```python
from build123d import *

# Parameters (mm, degrees)
MODEL_R             = 14.351
MODEL_R_2           = 2.413
BOSS_EXTRUDE1_DEPTH = 7.874
SKETCH17_R          = 2.0701
CUT_EXTRUDE1_DEPTH  = 8.874
SKETCH18_R          = 2.0193
CUT_EXTRUDE2_DEPTH  = 8.874


with BuildPart() as part:
    # Model → Boss-Extrude1 (new body)
    with BuildSketch(Plane.XY):
        with BuildLine():
            Line((127.809114586, 137.689660276), (-200.005250584, 313.419470721))
            ThreePointArc((-200.005250584, 313.419470721), (-219.438743814, 318.210854709), (-236.308771814, 307.439588539))
            Line((-236.308771814, 307.439588539), (-425.925316767, 28.829603592))
            ThreePointArc((-425.925316767, 28.829603592), (-430.312243104, 13.671313347), (-424.900993017, -1.152223962))
            Line((-424.900993017, -1.152223962), (-385.581467186, -51.204797614))
            ThreePointArc((-385.581467186, -51.204797614), (-376.711879358, -58.358090396), (-365.607528193, -60.913979882))
            Line((-365.607528193, -60.913979882), (-324.737451002, -60.913979882))
            ThreePointArc((-324.737451002, -60.913979882), (-318.798508014, -59.439796386), (-314.23831963, -55.359484793))
            Line((-314.23831963, -55.359484793), (-212.899365952, 93.541257838))
            ThreePointArc((-212.899365952, 93.541257838), (-203.778989185, 101.701881024), (-191.901103209, 104.650248016))
            Line((-191.901103209, 104.650248016), (48.661197018, 104.650248016))
            ThreePointArc((48.661197018, 104.650248016), (64.032332507, 99.471232012), (73.135172194, 86.046168785))
            Line((73.135172194, 86.046168785), (86.727013732, 37.098218434))
            ThreePointArc((86.727013732, 37.098218434), (106.362581421, 15.501750179), (127.326236921, 35.811553418))
            Line((127.326236921, 35.811553418), (140.807890588, 110.809453484))
            ThreePointArc((140.807890588, 110.809453484), (138.675228362, 126.361225539), (127.809114586, 137.689660276))
        make_face()
        with Locations((-323.775189267, -35.513979882)):
            Circle(MODEL_R, mode=Mode.SUBTRACT)
        with Locations((-399.975189267, 2.586020118)):
            Circle(MODEL_R, mode=Mode.SUBTRACT)
        with Locations((107.006236921, 23.111553418)):
            Circle(MODEL_R_2, mode=Mode.SUBTRACT)
        with Locations((94.306236921, 35.811553418)):
            Circle(MODEL_R_2, mode=Mode.SUBTRACT)
        Polygon((110.67241113, 42.161553418), (114.33858534, 35.811553418), (110.67241113, 29.461553418), (103.340062712, 29.461553418), (99.673888502, 35.811553418), (103.340062712, 42.161553418), (107.006236921, 42.161553418), align=None, mode=Mode.SUBTRACT)
        with Locations((119.706236921, 35.811553418)):
            Circle(MODEL_R_2, mode=Mode.SUBTRACT)
        with Locations((107.006236921, 48.511553418)):
            Circle(MODEL_R_2, mode=Mode.SUBTRACT)
        with Locations((-190.707148919, 138.516914683)):
            Circle(MODEL_R, mode=Mode.SUBTRACT)
        with Locations((-178.846696227, 264.756008796)):
            Circle(MODEL_R_2, mode=Mode.SUBTRACT)
        with Locations((-208.832932893, 283.437784316)):
            Circle(MODEL_R, mode=Mode.SUBTRACT)
        with Locations((-169.846303212, 281.545750473)):
            Circle(MODEL_R_2, mode=Mode.SUBTRACT)
        with Locations((-60.736830905, 201.457194342)):
            Circle(MODEL_R_2, mode=Mode.SUBTRACT)
        with Locations((-51.138479016, 217.912410568)):
            Circle(MODEL_R_2, mode=Mode.SUBTRACT)
    extrude(amount=BOSS_EXTRUDE1_DEPTH)

    # Sketch17 → Cut-Extrude1 (cut, through all)
    with BuildSketch(Plane(origin=(0, 0, 0), x_dir=(-1, 0, 0), z_dir=(0, 0, -1))):
        with Locations((138.53320591, 255.908211149)):
            Circle(SKETCH17_R)
        with Locations((147.519620664, 239.110983703)):
            Circle(SKETCH17_R)
        with Locations((125.123317403, 227.129097364)):
            Circle(SKETCH17_R)
        with Locations((116.136902649, 243.92632481)):
            Circle(SKETCH17_R)
    extrude(amount=-CUT_EXTRUDE1_DEPTH, mode=Mode.SUBTRACT)

    # Sketch18 → Cut-Extrude2 (cut, through all)
    with BuildSketch(Plane(origin=(0, 0, 0), x_dir=(-1, 0, 0), z_dir=(0, 0, -1))):
        with Locations((120.287453551, 146.062677987)):
            Circle(SKETCH18_R)
        with Locations((120.287453551, 127.012677987)):
            Circle(SKETCH18_R)
        with Locations((94.887453551, 127.012677987)):
            Circle(SKETCH18_R)
        with Locations((94.887453551, 146.062677987)):
            Circle(SKETCH18_R)
    extrude(amount=-CUT_EXTRUDE2_DEPTH, mode=Mode.SUBTRACT)


solid = part.part
```
Build history of the part. All positions in model axes, mm. A direction names the side the tool comes from. Coordinates: 2 decimals unless noted, no trailing zeros. Order: outer loops, then holes, each group sorted by start corner. A loop starts at its lowest first (then second) coordinate and runs counter-clockwise, first axis right, second up.
Item 1: Mould opens along Y. For faces 3 (the cylindrical face through (-210.701, 297.667, 3.882)), 4 (the flat face through (133.973, 72.786, 3.882)), 5 (the cylindrical face through (-310.52, -41.01, 3.88)), 6 (the flat face through (-149, 131, 7.874)) say: released by +Y, released by -Y, zero draft, split by the parting line, or undercut.
Filled in:
face 3: undercut
face 4: released by -Y
face 5: undercut
face 6: zero draft
Item 2: Drill centre lines: L1, parallel to Y at x = -178.5, z = 3.5; L2, parallel to X at y = 125.5, z = 2; L3, parallel to Y at x = -392, z = 6.5. Where is each one in solid material? Low to high.
Filled in:
L1: y = 104.65 to 130.97, 146.06 to 262.37, 267.14 to 301.89
L2: x = -360.13 to -196.75, -184.66 to -121.63, -118.95 to -96.23, -93.55 to 139.07
L3: y = -43.03 to -9.34, 14.52 to 78.68
Item 3: Saw through at B-B on x = -347. List the corners of the cut face in (y, z), then the cut area to 3 significant figures.
Filled in:
outline: (-60.91, 0) - (144.8, 0) - (144.8, 7.87) - (-60.91, 7.87) - close
area: 1,620 mm2
Item 4: Saw through at A-A on y = 57.5. List the corners of the cut face in (x, z).
Filled in:
outline: (-406.41, 0) - (-237.43, 0) - (-237.43, 7.87) - (-406.41, 7.87) - close; (81.06, 0) - (131.22, 0) - (131.22, 7.87) - (81.06, 7.87) - close
Item 5: Saw through at D-D on x = -38. List the corners of the cut face in (y, z).
Filled in:
outline: (104.65, 0) - (226.57, 0) - (226.57, 7.87) - (104.65, 7.87) - close
Item 6: Drop flat-ended pins along their axis: pin 1 Ø4 at (x, y) = (94.31, 35.81) entering from +Z; pin 2 Ø3 at (y, z) = (76, 7) entering from -X; pin 3 Ø1 at (x, z) = (-55.5, 3) entering from +Y; pin 4 Ø4 at (x, z) = (-49, 5) entering from -Y. Give the stop position or say it passes through.
Filled in:
pin 1: passes through
pin 2: stops at x = -394.84
pin 3: stops at y = 236.22
pin 4: stops at y = 104.65
Item 7: Tool access for faces 1 (the cylindrical face through (-203.93, 101.62, 3.88)), 2 (the cylindrical face through (-219.154, 318.256, 3.882)): list every direction of +Z, -Z, +X, -X, +Y, -Y with a clear straight run to the whole face (end or side of a thin tool).
Filled in:
face 1: +Z, -Z, -Y
face 2: +Z, -Z, +Y
Item 8: Saw through at C-C on z = 4.25. State how many separate pieces and enclosed holes the cut face has, then the cut area to 3 significant figures.
Filled in:
separate pieces: 1
enclosed holes: 21
area: 87,100 mm2
